```python
from build123d import *

# Parameters (mm, degrees)
BOSS_EXTRUDE1_DEPTH = 6.35


with BuildPart() as part:
    # Sketch1 → Boss-Extrude1 (new body)
    with BuildSketch(Plane.XY):
        with BuildLine():
            Line((10.705286018, 0), (18.039645204, 27.372201124))
            ThreePointArc((18.039645204, 27.372201124), (27.372201124, 32.760354796), (32.760354796, 23.427798876))
            Line((32.760354796, 23.427798876), (26.482895007, 0))
            Line((26.482895007, 0), (50.8, 0))
            Line((50.8, 0), (50.8, 76.2))
            Line((50.8, 76.2), (0, 76.2))
            Line((0, 76.2), (0, 0))
            Line((0, 0), (10.705286018, 0))
        make_face()
    extrude(amount=BOSS_EXTRUDE1_DEPTH)


solid = part.part
```
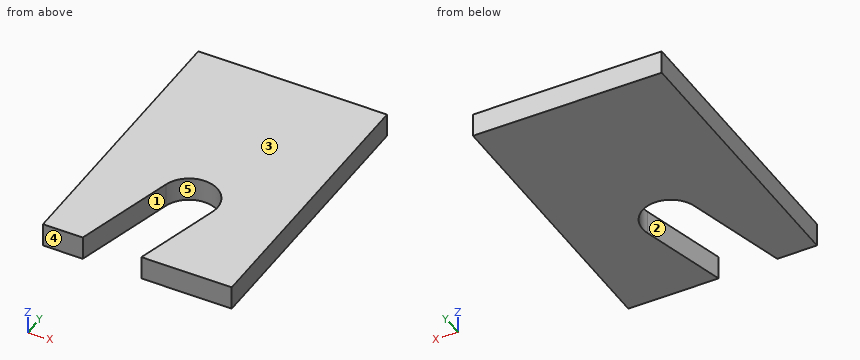
Source: CAD feature listing. Evaluate the final solid. Frame: model axes, mm. Face numbers are marked on the shaded views. A direction names the side the tool comes from. Give positions to 0.01 mm unless a question says otherwise; leave off trailing zeros. Write each loop counter-clockwise with the first axis right and the second up, starting at its lowest first coordinate (ties: lowest second). Pieces come first, ordered by that corner, then holes. Notation, with made-up numbers: (52.25, 10) - (82.25, 10) arc R25 cw to (82.25, 49) - close; hole circle Ø6 at (-32.75, -24.75). An arc over 180 degrees is marked (long way). One line per item, written item: value. Start each with the question number.
Q1. Section query B-B, the plane z = 2.25. Return the cut outline in (x, y), then the cut area to 3 significant figures.
Q2. Draft query along X for the marked faces 4 and 5. Return one class per face: +X half, -X half, draft (parallel to the pull), parting line (faces both ways), or undercut.
Q3. Section query D-D, the plane x = 19. Return the cut outline in (y, z), then the cut area to 3 significant figures.
Q4. Section query A-A, the plane y = 25.4. Return the cut outline in (x, z), then the cut area to 3 significant figures.
Q5. Set-up query: the marked faces 1, 2 and 3. Return all of +Z, -Z, +X, -X, +Y, -Y with unobstructed straight access to the full face (end or side cutting, diameter ignored); none if empty.
Q6. Material intervals for probe 1 along X at (y, z) = (32, 5.25); probe 2 along X at (y, z) = (9.5, 5.5); probe 3 along Y at (x, z) = (25, 5.75), sorted ascending. Write a range as from..to.
Q7. Section query C-C, the plane x = 30. Return the cut outline in (y, z).
Answer:
1. outline: (0, 0) - (10.71, 0) - (18.04, 27.37) arc R7.62 cw to (32.76, 23.43) - (26.48, 0) - (50.8, 0) - (50.8, 76.2) - (0, 76.2) - close
1. area: 3,380 mm2
2. face 4: draft
2. face 5: undercut
3. outline: (29.54, 0) - (76.2, 0) - (76.2, 6.35) - (29.54, 6.35) - close
3. area: 296 mm2
4. outline: (0, 0) - (17.51, 0) - (17.51, 6.35) - (0, 6.35) - close; (33.02, 0) - (50.8, 0) - (50.8, 6.35) - (33.02, 6.35) - close
4. area: 224 mm2
5. face 1: +Z, -Z, -Y
5. face 2: +Z, -Z
5. face 3: +Z, +X, -X, +Y, -Y
6. probe 1: x = 0..21.59, 29.21..50.8
6. probe 2: x = 0..13.25, 29.03..50.8
6. probe 3: y = 33.01..76.2
7. outline: (0, 0) - (13.13, 0) - (13.13, 6.35) - (0, 6.35) - close; (31.47, 0) - (76.2, 0) - (76.2, 6.35) - (31.47, 6.35) - close
